Verification items for the finished model (mm, model axes). Give positions to 0.01 mm unless a question says otherwise; leave off trailing zeros. Loops run counter-clockwise (first coordinate to the right, second up) from the corner with the lowest first, then second, coordinate; pieces in that order, holes last. Notation, with made-up numbers: (2.5, 75) - (58.5, 75) arc R23 ccw to (58.5, 94) - close; hole circle Ø11 at (77.5, 57). An arc over 180 degrees is marked (long way). Put each result on its own line as item: value. Start each with the question number.
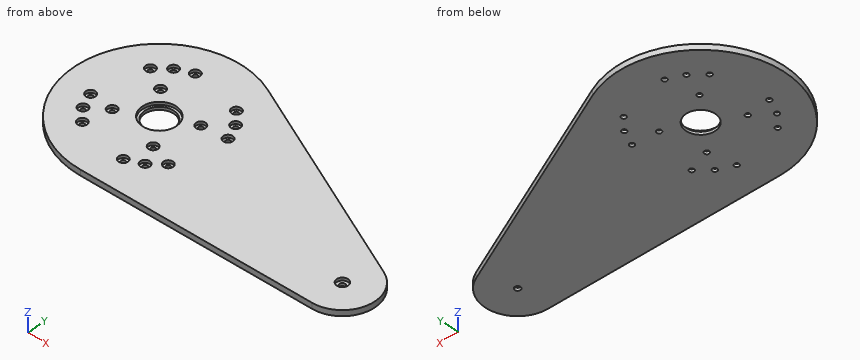
```python
from build123d import *

# Parameters (mm, degrees)
SKETCH_R              = 3
SKETCH_R_2            = 15.5
PAD_DEPTH             = 6
SKETCH001_R           = 2.5
POCKET_DEPTH          = 10
POLARPATTERN_COUNT    = 4
SKETCH002_R           = 5
POCKET001_DEPTH       = 3
POLARPATTERN001_COUNT = 4
SKETCH003_R           = 6
POCKET002_DEPTH       = 3
SKETCH004_R           = 18
POCKET003_DEPTH       = 3
SKETCH010_R           = 2.5
POCKET007_DEPTH       = 6
SKETCH011_R           = 5
POCKET008_DEPTH       = 3
POLARPATTERN004_COUNT = 4
SKETCH012_R           = 2.5
POCKET009_DEPTH       = 6
SKETCH013_R           = 5
POCKET010_DEPTH       = 3
CLONE_PLACEMENT_ANGLE = 13


with BuildPart() as part:
    # Sketch → Pad (new body)
    with BuildSketch(Plane.XY):
        with BuildLine():
            ThreePointArc((19.98, 87.7542), (-90, 0), (19.98, -87.7542))
            Line((19.98, -87.7542), (257.659, -33.63911))
            ThreePointArc((257.659, -33.63911), (284.5, 0), (257.659, 33.63911))
            Line((19.98, 87.7542), (257.659, 33.63911))
        make_face()
        with Locations((250, 0)):
            Circle(SKETCH_R, mode=Mode.SUBTRACT)
        Circle(SKETCH_R_2, mode=Mode.SUBTRACT)
    extrude(amount=PAD_DEPTH)

    # Sketch001 (on Face8 of Pad) → Pocket (cut)
    with BuildSketch(Plane.XY.offset(6)):
        with Locations((42.4248, 42.428014)):
            Circle(SKETCH001_R)
    pocket = extrude(amount=-POCKET_DEPTH, mode=Mode.SUBTRACT)

    # PolarPattern: Pocket ×4 about axis
    polarpattern_axis = Axis((0, 0, 6), (0, 0, 1))
    for i in range(1, POLARPATTERN_COUNT):
        add(pocket.rotate(polarpattern_axis, i * 360 / POLARPATTERN_COUNT), mode=Mode.SUBTRACT)

    # Sketch002 (on Face5 of PolarPattern) → Pocket001 (cut)
    with BuildSketch(Plane.XY.offset(6)):
        with Locations((-42.428014, 42.4248)):
            Circle(SKETCH002_R)
    pocket001 = extrude(amount=-POCKET001_DEPTH, mode=Mode.SUBTRACT)

    # PolarPattern001: Pocket001 ×4 about axis
    polarpattern001_axis = Axis((0, 0, 6), (0, 0, 1))
    for i in range(1, POLARPATTERN001_COUNT):
        add(pocket001.rotate(polarpattern001_axis, i * 360 / POLARPATTERN001_COUNT), mode=Mode.SUBTRACT)

    # Sketch003 (on Face5 of PolarPattern001) → Pocket002 (cut)
    with BuildSketch(Plane.XY.offset(6)):
        with Locations((250, 0)):
            Circle(SKETCH003_R)
    extrude(amount=-POCKET002_DEPTH, mode=Mode.SUBTRACT)

    # Sketch004 (on Face5 of Pocket002) → Pocket003 (cut)
    with BuildSketch(Plane.XY.offset(6)):
        Circle(SKETCH004_R)
    extrude(amount=-POCKET003_DEPTH, mode=Mode.SUBTRACT)

    # Sketch010 (on Face5 of Pocket003) → Pocket007 (cut)
    with BuildSketch(Plane.XY.offset(6)):
        with Locations((53, 28)):
            Circle(SKETCH010_R)
        with Locations((53, -28)):
            Circle(SKETCH010_R)
    pocket007 = extrude(amount=-POCKET007_DEPTH, mode=Mode.SUBTRACT)

    # Sketch011 (on Face5 of Pocket007) → Pocket008 (cut)
    with BuildSketch(Plane.XY.offset(6)):
        with Locations((53, 28)):
            Circle(SKETCH011_R)
        with Locations((53, -28)):
            Circle(SKETCH011_R)
    pocket008 = extrude(amount=-POCKET008_DEPTH, mode=Mode.SUBTRACT)

    # PolarPattern004: Pocket007, Pocket008 ×4 about axis
    polarpattern004_axis = Axis((0, 0, 6), (0, 0, 1))
    for i in range(1, POLARPATTERN004_COUNT):
        add(pocket007.rotate(polarpattern004_axis, i * 360 / POLARPATTERN004_COUNT), mode=Mode.SUBTRACT)
        add(pocket008.rotate(polarpattern004_axis, i * 360 / POLARPATTERN004_COUNT), mode=Mode.SUBTRACT)

    # Sketch012 (on Face5 of PolarPattern004) → Pocket009 (cut)
    with BuildSketch(Plane.XY.offset(6)):
        with Locations((28, -25)):
            Circle(SKETCH012_R)
        with Locations((27.5, 20)):
            Circle(SKETCH012_R)
    pocket009 = extrude(amount=-POCKET009_DEPTH, mode=Mode.SUBTRACT)

    # Sketch013 (on Face5 of Pocket009) → Pocket010 (cut)
    with BuildSketch(Plane.XY.offset(6)):
        with Locations((27.5, 20)):
            Circle(SKETCH013_R)
        with Locations((28, -25)):
            Circle(SKETCH013_R)
    pocket010 = extrude(amount=-POCKET010_DEPTH, mode=Mode.SUBTRACT)

    # Mirrored: Pocket010, Pocket009 across Sketch013 V_Axis
    add(pocket010.mirror(Plane(origin=(0, 0, 6), x_dir=(0, 0, 1), z_dir=(1, 0, 0))), mode=Mode.SUBTRACT)
    add(pocket009.mirror(Plane(origin=(0, 0, 6), x_dir=(0, 0, 1), z_dir=(1, 0, 0))), mode=Mode.SUBTRACT)


with BuildPart() as part_1:
    # Clone placement: moved
    add(part.part.moved(Location((105, 104.973082, -6))).rotate(Axis((105, 104.973082, -6), (0, 0, -1)), CLONE_PLACEMENT_ANGLE))


solid = part_1.part
```
1) Section check B-B, the plane x = 110. Enter the section's corners in (y, z).
2) Section check D-D, the plane x = 199.5. Enter the section's corners in (y, z).
3) Section check C-C, the plane y = 179. Enter the section's corners in (x, z).
4) Scan lines: line 1 along X through (y, z) = (135, -1.6); line 2 along Y through (x, z) = (105, -1.65); line 3 along X through (y, z) = (93, -0.4). Record each from-to range of solid material in increasing order. Write a range as from..to.
5) Depth check by flat-ended pin: P1, Ø2, axis at x = 105.5, y = 88.5, coming from the +Z side; P2, Ø1.5, axis at y = 92, z = -1.5, coming from the +X side. Enter the tip coordinate at first touch or a pass-through.
6) Section check A-A, the plane z = -4.7. State how many separate pieces and enclosed holes the cut face has, plus the area to 3 significant figures.
Results are:
1. outline: (14.96, -6) - (90.3, -6) - (90.3, -3) - (87.68, -3) - (87.68, 0) - (14.96, 0) - close; (119.64, -6) - (194.83, -6) - (194.83, 0) - (122.26, 0) - (122.26, -3) - (119.64, -3) - close
2. outline: (14.69, -6) - (159.22, -6) - (159.22, 0) - (14.69, 0) - close
3. outline: (53.81, -6) - (158.64, -6) - (158.64, 0) - (53.81, 0) - close
4. line 1: x = 20.16..80.24, 85.16..151.21, 160.56..249.55
4. line 2: y = 14.97..86.97, 122.97..194.97
4. line 3: x = 15.8..43.38, 50.74..91.56, 118.44..336.33
5. P1: stops at z = -3
5. P2: stops at x = 339.94
6. separate pieces: 1
6. enclosed holes: 18
6. area: 45,400 mm2
